from build123d import *

# Parameters (mm, degrees)
F0_W      = 76.2
F0_H      = 44.45
F1_DEPTH  = 25.4
F2_W      = 25.4
F2_H      = 25.4
F3_DEPTH  = 31.75
F4_R      = 6.35
F5_DEPTH  = 25.4
F6_R      = 6.35
F7_DEPTH  = 25.4
F9_DEPTH  = 25.4
F11_DEPTH = 25.4
F13_DEPTH = 25.4


with BuildPart() as f1:
    # F0 (on Front) → F1 (new body)
    with BuildSketch(Plane.XZ):
        with Locations((38.1, 22.225)):
            Rectangle(F0_W, F0_H)
    extrude(amount=F1_DEPTH)

    # F2 (on face) → F3 (cut)
    with BuildSketch(Plane.XY.offset(44.45)):
        with Locations((63.5, -12.7)):
            Rectangle(F2_W, F2_H)
        with Locations((12.7, -12.7)):
            Rectangle(F2_W, F2_H)
    extrude(amount=-F3_DEPTH, mode=Mode.SUBTRACT)

    # F4 (on face) → F5 (cut)
    with BuildSketch(Plane.XY.offset(12.7)):
        with Locations((12.7, -12.7)):
            Circle(F4_R)
        with Locations((63.5, -12.7)):
            Circle(F4_R)
    extrude(amount=-F5_DEPTH, mode=Mode.SUBTRACT)

    # F6 (on face) → F7 (cut)
    with BuildSketch(Plane.YZ.offset(50.8)):
        with Locations((-12.7, 31.75)):
            Circle(F6_R)
    extrude(amount=-F7_DEPTH, mode=Mode.SUBTRACT)

    # F8 (on face) → F9 (cut)
    with BuildSketch(Plane.XY.offset(12.7)):
        with BuildLine():
            ThreePointArc((69.85, 0), (74.5240316571, -5.6004841714), (76.2, -12.7))
            Line((76.2, -12.7), (76.2, 0))
            Line((76.2, 0), (69.85, 0))
        make_face()
        with BuildLine():
            ThreePointArc((76.2, -12.7), (74.5240316571, -19.7995158286), (69.85, -25.4))
            Line((69.85, -25.4), (76.2, -25.4))
            Line((76.2, -25.4), (76.2, -12.7))
        make_face()
    extrude(amount=-F9_DEPTH, mode=Mode.SUBTRACT)

    # F10 (on face) → F11 (cut)
    with BuildSketch(Plane.XY.offset(12.7)):
        with BuildLine():
            ThreePointArc((0, -12.6999999584), (1.6759683522, -5.6004841529), (6.35, 0))
            Line((6.35, 0), (0, 0))
            Line((0, 0), (0, -12.6999999584))
        make_face()
        with BuildLine():
            ThreePointArc((6.35, -25.4), (1.6759683336, -19.79951581), (0, -12.6999999584))
            Line((0, -12.6999999584), (0, -25.4))
            Line((0, -25.4), (6.35, -25.4))
        make_face()
    extrude(amount=-F11_DEPTH, mode=Mode.SUBTRACT)

    # F12 (on face) → F13 (cut)
    with BuildSketch(Plane.YZ.offset(50.8)):
        with BuildLine():
            ThreePointArc((-25.4, 31.75), (-21.6802561211, 40.7302561211), (-12.7, 44.45))
            Line((-12.7, 44.45), (-25.4, 44.45))
            Line((-25.4, 44.45), (-25.4, 31.75))
        make_face()
        with BuildLine():
            ThreePointArc((-12.7, 44.45), (-3.7197438789, 40.7302561211), (0, 31.75))
            Line((0, 31.75), (0, 44.45))
            Line((0, 44.45), (-12.7, 44.45))
        make_face()
    extrude(amount=-F13_DEPTH, mode=Mode.SUBTRACT)


solid = f1.part
Design review of the part built by this model. Coordinates are the model's own, in mm. A direction names the side the tool comes from. Coordinates: 2 decimals unless noted, no trailing zeros. Write each loop counter-clockwise with the first axis right and the second up, starting at its lowest first coordinate (ties: lowest second). Pieces come first, ordered by that corner, then holes. Notation, with made-up numbers: (10, -8.75) - (30, -8.75) arc R21 ccw to (30, 20.25) - close; hole circle Ø6 at (0, 35). An arc over 180 degrees is marked (long way). Use one line per item in the form item = value.
Q1. Consider section C-C (y = -18). Write out the cut boundary in (x, z).
Taken from the geometry:
outline = (0.91, 0) - (9.2, 0) - (9.2, 12.7) - (0.91, 12.7) - close; (16.2, 0) - (60, 0) - (60, 12.7) - (50.8, 12.7) - (50.8, 28.25) - (25.4, 28.25) - (25.4, 12.7) - (16.2, 12.7) - close; (25.4, 35.25) - (50.8, 35.25) - (50.8, 43.29) - (25.4, 43.29) - close; (67, 0) - (75.29, 0) - (75.29, 12.7) - (67, 12.7) - close
Q2. Consider section A-A (x = 12.7). Write out the cut boundary in (y, z), plus the area to 3 significant figures.
Taken from the geometry:
outline = (-25.4, 0) - (-19.05, 0) - (-19.05, 12.7) - (-25.4, 12.7) - close; (-6.35, 0) - (0, 0) - (0, 12.7) - (-6.35, 12.7) - close
area = 161 mm^2
Q3. The part is to be moulded in two halves that separate along X. For faces 4 (the flat face through (25.4, -13, 25)), 5 (the flat face through (38, 0, 13)), 6 (the cylindrical face through (7.66, -16.56, 6.44)), say which applies: +X half, -X half, draft (parallel to the pull), parting line (faces both ways), or undercut.
Taken from the geometry:
face_4 = -X half
face_5 = draft
face_6 = undercut
Q4. Insertion check: pin 1 Ø8 at (y, z) = (-6.5, 13.5) entering from -X; pin 2 Ø10 at (x, y) = (40.5, -4.5) entering from +Z; pin 3 Ø14.5 at (y, z) = (-12.7, 31.75) entering from -X. Each pin has a flat end and moves straight along its axis. Give the tip position at first contact, or say it passes through.
Taken from the geometry:
pin_1 = 0.16
pin_2 = 44.04
pin_3 = 25.4
Q5. Machinability: for faces 1 (the flat face through (9.7, -6.9, 12.7)), 2 (the flat face through (38, -25.4, 13)), 3 (the flat face through (50.8, -13, 25)), which of the approach directions +Z, -Z, +X, -X, +Y, -Y give a long, thin tool a straight path to every point of the face, cutting with its end or side? Answer none if there is none.
Taken from the geometry:
face_1 = +Z, -X, +Y, -Y
face_2 = +Z, -Z, +X, -X, -Y
face_3 = +Z, +X, +Y, -Y
Q6. Consider section B-B (z = 11). Write out the cut boundary in (x, y) (3 decimals), plus the area to 4 significant figures.
Taken from the geometry:
outline = (6.35, -25.4) - (69.85, -25.4) arc R15.875 ccw to (69.85, 0) - (6.35, 0) arc R15.875 ccw to start; hole circle Ø12.7 at (12.7, -12.7); hole circle Ø12.7 at (63.5, -12.7)
area = 1,585 mm^2
Q7. For probe 1 along X at (y, z) = (-12.5, 10); probe 2 along Z at (x, y) = (33, -12.7); probe 3 along X at (y, z) = (-15, 11.5), list the stretches that pass through material, from the lowest coordinate up.
Taken from the geometry:
probe_1 = 0 to 6.35, 19.05 to 57.15, 69.85 to 76.2
probe_2 = 0 to 25.4, 38.1 to 44.45
probe_3 = 0.17 to 6.78, 18.62 to 57.58, 69.42 to 76.03
Q8. Consider section D-D (z = 33.5). Write out the cut boundary in (x, y).
Taken from the geometry:
outline = (25.4, -25.28) - (50.8, -25.28) - (50.8, -18.8) - (25.4, -18.8) - close; (25.4, -6.6) - (50.8, -6.6) - (50.8, -0.12) - (25.4, -0.12) - close
